```python
from build123d import *

# Parameters (mm, degrees)
BOSS_EXTRUDE1_DEPTH      = 1
SKETCH2_R                = 0.26
BOSS_EXTRUDE2_DEPTH      = 10
BOSS_EXTRUDE2_DEPTH_BACK = 1.1
CUT_EXTRUDE1_DEPTH       = 0.01
FILLET1_R                = 0.1


with BuildPart() as part:
    # Sketch1 → Boss-Extrude1 (new body)
    with BuildSketch(Plane(origin=(0, 0, 0), x_dir=(1, 0, 0), z_dir=(0, 1, 0))):
        with BuildLine():
            Line((-1.9, 1.251249376), (-1.9, -1.251249376))
            ThreePointArc((-1.9, -1.251249376), (0, -2.275), (1.9, -1.251249376))
            Line((1.9, -1.251249376), (1.9, 1.251249376))
            ThreePointArc((1.9, 1.251249376), (0, 2.275), (-1.9, 1.251249376))
        make_face()
    extrude(amount=BOSS_EXTRUDE1_DEPTH)

    # Sketch2 → Boss-Extrude2 (add, two sides)
    with BuildSketch(Plane(origin=(0, 1, 0), x_dir=(1, 0, 0), z_dir=(0, 1, 0))) as boss_extrude2_sk:
        with Locations((0, 1.295)):
            Circle(SKETCH2_R)
        with Locations((0, -1.295)):
            Circle(SKETCH2_R)
    extrude(amount=BOSS_EXTRUDE2_DEPTH)
    extrude(boss_extrude2_sk.sketch, amount=-BOSS_EXTRUDE2_DEPTH_BACK)

    # Sketch4 → Cut-Extrude1 (cut)
    with BuildSketch(Plane.XZ):
        with BuildLine():
            Line((1.9, -1.251249376), (1.9, 1.251249376))
            ThreePointArc((1.9, 1.251249376), (0, 2.275), (-1.9, 1.251249376))
            Line((-1.9, 1.251249376), (-1.9, -1.251249376))
            ThreePointArc((-1.9, -1.251249376), (0, -2.275), (1.9, -1.251249376))
        make_face()
        with BuildLine():
            Line((-1.4, 1.091157642), (-1.4, -1.091157642))
            ThreePointArc((-1.4, -1.091157642), (0, -1.775), (1.4, -1.091157642))
            Line((1.4, -1.091157642), (1.4, 1.091157642))
            ThreePointArc((1.4, 1.091157642), (1.375341403, 1.122078885), (1.35, 1.152443057))
            Line((1.35, 1.152443057), (1.35, -1))
            ThreePointArc((1.35, -1), (1.2, -1.15), (1.05, -1))
            Line((1.05, -1), (1.05, 0.9))
            ThreePointArc((1.05, 0.9), (0.9, 1.05), (0.75, 0.9))
            Line((0.75, 0.9), (0.75, -0.9))
            ThreePointArc((0.75, -0.9), (0.6, -1.05), (0.45, -0.9))
            Line((0.45, -0.9), (0.45, 0.7))
            ThreePointArc((0.45, 0.7), (0.3, 0.85), (0.15, 0.7))
            Line((0.15, 0.7), (0.15, -0.75))
            ThreePointArc((0.15, -0.75), (0, -0.9), (-0.15, -0.75))
            Line((-0.15, -0.75), (-0.15, 0.7))
            ThreePointArc((-0.15, 0.7), (-0.3, 0.85), (-0.45, 0.7))
            Line((-0.45, 0.7), (-0.45, -0.9))
            ThreePointArc((-0.45, -0.9), (-0.6, -1.05), (-0.75, -0.9))
            Line((-0.75, -0.9), (-0.75, 0.9))
            ThreePointArc((-0.75, 0.9), (-0.9, 1.05), (-1.05, 0.9))
            Line((-1.05, 0.9), (-1.05, -1))
            ThreePointArc((-1.05, -1), (-1.2, -1.15), (-1.35, -1))
            Line((-1.35, -1), (-1.35, 1.152443057))
            ThreePointArc((-1.35, 1.152443057), (-1.375341403, 1.122078885), (-1.4, 1.091157642))
        make_face(mode=Mode.SUBTRACT)
        with BuildLine():
            Line((1.25, 1.152443057), (1.25, -1))
            ThreePointArc((1.25, -1), (1.2, -1.05), (1.15, -1))
            Line((1.15, -1), (1.15, 0.9))
            ThreePointArc((1.15, 0.9), (0.9, 1.15), (0.65, 0.9))
            Line((0.65, 0.9), (0.65, -0.9))
            ThreePointArc((0.65, -0.9), (0.6, -0.95), (0.55, -0.9))
            Line((0.55, -0.9), (0.55, 0.7))
            ThreePointArc((0.55, 0.7), (0.3, 0.95), (0.05, 0.7))
            Line((0.05, 0.7), (0.05, -0.75))
            ThreePointArc((0.05, -0.75), (0.035355339, -0.785355339), (0, -0.8))
            ThreePointArc((0, -0.8), (-0.035355339, -0.785355339), (-0.05, -0.75))
            Line((-0.05, -0.75), (-0.05, 0.7))
            ThreePointArc((-0.05, 0.7), (-0.3, 0.95), (-0.55, 0.7))
            Line((-0.55, 0.7), (-0.55, -0.9))
            ThreePointArc((-0.55, -0.9), (-0.6, -0.95), (-0.65, -0.9))
            Line((-0.65, -0.9), (-0.65, 0.9))
            ThreePointArc((-0.65, 0.9), (-0.9, 1.15), (-1.15, 0.9))
            Line((-1.15, 0.9), (-1.15, -1))
            ThreePointArc((-1.15, -1), (-1.2, -1.05), (-1.25, -1))
            Line((-1.25, -1), (-1.25, 1.152443057))
            Line((-1.25, 1.152443057), (-1.25, 1.260208316))
            ThreePointArc((-1.25, 1.260208316), (0, 1.775), (1.25, 1.260208316))
            Line((1.25, 1.260208316), (1.25, 1.152443057))
        make_face(mode=Mode.SUBTRACT)
    extrude(amount=-CUT_EXTRUDE1_DEPTH, mode=Mode.SUBTRACT)

    # Fillet1
    fillet1_edges = [part.edges().sort_by_distance(p)[0] for p in [
        (0, 1, 2.275),
        (1.9, 1, 0),
        (0, 1, -2.275),
        (0, 0.01, -2.275),
        (-1.9, 0.01, 0),
        (0, 0.01, 2.275),
        (1.9, 0.01, 0),
        (-1.9, 1, 0),
        (1.9, 0.505, -1.251249376),
        (1.9, 0.505, 1.251249376),
        (-1.9, 0.505, 1.251249376),
        (-1.9, 0.505, -1.251249376),
    ]]
    fillet(fillet1_edges, radius=FILLET1_R)


solid = part.part
```
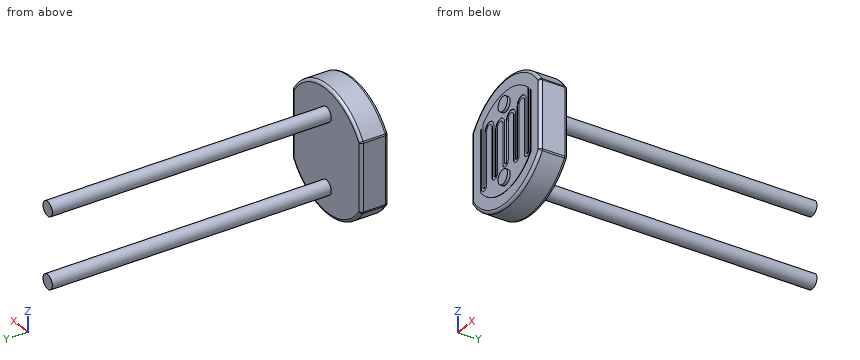
Geometry: final body of the model. Coordinates: model frame, mm. Round coordinates to 2 decimals unless told otherwise and drop trailing zeros. Write each loop counter-clockwise with the first axis right and the second up, starting at its lowest first coordinate (ties: lowest second). Pieces come first, ordered by that corner, then holes. Notation, with made-up numbers: (75, 0) -> (115, 0) arc R22 cw to (115, 33) -> close; hole circle Ø7 at (-7.75, 77). An arc over 180 degrees is marked (long way). Use CSV: the item, a comma, the result in double quotes. Start each with the question number.
Q1. Line query: L1, parallel to Y at x = 0.25, z = -1.45; L2, parallel to X at y = 4.75, z = -1.3; L3, parallel to X at y = 2, z = 1.1. Output: solid intervals per line, ascending.
Q2. Section B-B (y = 9). Return loops of the section in (x, z) (3 decimals).
Q3. Section A-A (y = 0.75). Return loops of the section in (x, z) (3 decimals).
Result sheet:
1,L1,"0 to 1"
1,L2,"-0.26 to 0.26"
1,L3,"-0.17 to 0.17"
2,outline,"circle Ø0.52 at (0, -1.295); circle Ø0.52 at (0, 1.295)"
3,outline,"(-1.9, -1.221) arc R0.1 ccw to (-1.883, -1.277) arc R2.275 ccw to (1.883, -1.277) arc R0.1 ccw to (1.9, -1.221) -> (1.9, 1.221) arc R0.1 ccw to (1.883, 1.277) arc R2.275 ccw to (-1.883, 1.277) arc R0.1 ccw to (-1.9, 1.221) -> close"
